CAD build for the part. Positions are in the model's coordinates, mm. Coordinates: 2 decimals unless noted, no trailing zeros. Order: outer loops, then holes, each group sorted by start corner. A loop starts at its lowest first (then second) coordinate and runs counter-clockwise, first axis right, second up.
from build123d import *

# Parameters (mm, degrees)
SKETCH1_R               = 50.8
SKETCH1_R_2             = 48.26
BOSS_EXTRUDE1_DEPTH     = 787.4
CUT_EXTRUDE1_DEPTH      = 791.670626747
CUT_EXTRUDE1_DEPTH_BACK = 791.670626747
SKETCH2_W               = 10.16
SKETCH2_H               = 112.776
CUT_EXTRUDE2_DEPTH      = 791.670626747
CUT_EXTRUDE2_DEPTH_BACK = 791.670626747
SKETCH3_W               = 10.16
SKETCH3_H               = 112.776


with BuildPart() as part:
    # Sketch1 → Boss-Extrude1 (new body)
    with BuildSketch(Plane(origin=(0, 0, 0), x_dir=(1, 0, 0), z_dir=(0, 1, 0))):
        with Locations(Location((0, 0, 0), (0, 0, 270))):
            Circle(SKETCH1_R)
        with Locations(Location((0, 0, 0), (0, 0, 270))):
            Circle(SKETCH1_R_2, mode=Mode.SUBTRACT)
    extrude(amount=BOSS_EXTRUDE1_DEPTH)

    # Sketch2 → Cut-Extrude1 (cut, two sides: drawn at the far end of the back side and taken through both)
    with BuildSketch(Plane.XY.offset(-CUT_EXTRUDE1_DEPTH_BACK)):
        with Locations((0, 81.788)):
            Rectangle(SKETCH2_W, SKETCH2_H)
    extrude(amount=CUT_EXTRUDE1_DEPTH + CUT_EXTRUDE1_DEPTH_BACK, mode=Mode.SUBTRACT)

    # Sketch3 → Cut-Extrude2 (cut, two sides: drawn at the far end of the back side and taken through both)
    with BuildSketch(Plane(origin=(0, 0, 0), x_dir=(0, 0, -1), z_dir=(1, 0, 0)).offset(-CUT_EXTRUDE2_DEPTH_BACK)):
        with Locations((0, 81.788)):
            Rectangle(SKETCH3_W, SKETCH3_H)
    extrude(amount=CUT_EXTRUDE2_DEPTH + CUT_EXTRUDE2_DEPTH_BACK, mode=Mode.SUBTRACT)


solid = part.part
1) Slice it at C-C (z = -30.5). List the corners of the cut face in (x, y) (3 decimals), plus the area to 3 significant figures.
2) Slice it at B-B (x = 26). List the corners of the cut face in (y, z), plus the area to 3 significant figures.
3) Drill centre lines: probe 1 along X at (y, z) = (184, 0); probe 2 along Z at (x, y) = (4, 632.5); probe 3 along X at (y, z) = (150, -1). Where is each one in solid material? Low to high.
4) Slice it at D-D (y = 355.5). List the corners of the cut face in (x, z).
5) Two-plate mould, pull along Z, no slides. Class faces 1 (the cylindrical face through (14.5, 388.19, 46.03)), 2 (the flat face through (-19, 0, 45)), 3 (the cylindrical face through (15.259, 388.188, 48.454)): released by +Z, released by -Z, zero draft, split by the parting line, or undercut.
6) Pin check, flat tips, straight feed: P1, Ø3, axis at y = 231, z = 28, coming from the +X side; P2, Ø1, axis at x = 29.5, y = 655.5, coming from the -Z side; P3, Ø1.5, axis at x = 35, y = 453.5, coming from the -Z side; P4, Ø1.4, axis at x = -2.5, z = 50, coming from the -Y side. Stop position of each tip, or through.
7) Slice it at A-A (y = 118.5). List the corners of the cut face in (x, z).
Worked out:
1. outline: (-40.625, 0) - (-37.4, 0) - (-37.4, 787.4) - (-40.625, 787.4) - close; (37.4, 0) - (40.625, 0) - (40.625, 787.4) - (37.4, 787.4) - close
1. area: 5,080 mm2
2. outline: (0, -43.64) - (787.4, -43.64) - (787.4, -40.66) - (0, -40.66) - close; (0, 40.66) - (787.4, 40.66) - (787.4, 43.64) - (0, 43.64) - close
2. area: 4,700 mm2
3. probe 1: x = -50.8 to -48.26, 48.26 to 50.8
3. probe 2: z = -50.64 to -48.09, 48.09 to 50.64
3. probe 3: x = -50.79 to -48.25, 48.25 to 50.79
4. outline: circle Ø101.6 at (0, 0); hole circle Ø96.52 at (0, 0)
5. face 1: undercut
5. face 2: zero draft
5. face 3: split by the parting line
6. P1: stops at x = 43.34
6. P2: stops at z = -41.71
6. P3: stops at z = -37.52
6. P4: stops at y = 0
7. outline: (-50.55, -5.08) arc R50.8 ccw to (-5.08, -50.55) - (-5.08, -47.99) arc R48.26 cw to (-47.99, -5.08) - close; (-50.55, 5.08) - (-47.99, 5.08) arc R48.26 cw to (-5.08, 47.99) - (-5.08, 50.55) arc R50.8 ccw to start; (5.08, -50.55) arc R50.8 ccw to (50.55, -5.08) - (47.99, -5.08) arc R48.26 cw to (5.08, -47.99) - close; (5.08, 47.99) arc R48.26 cw to (47.99, 5.08) - (50.55, 5.08) arc R50.8 ccw to (5.08, 50.55) - close
